Verification items for the finished model (mm, model axes). Coordinates: 2 decimals unless noted, no trailing zeros. Order: outer loops, then holes, each group sorted by start corner. A loop starts at its lowest first (then second) coordinate and runs counter-clockwise, first axis right, second up. Notation, with made-up numbers: M -23,25.25 L 17,25.25 A25 cw 17,56.25 Z; hole C -29,44.5 d8. An arc over 180 degrees is marked long. Return JSON: item names as keys, results as strings. Group by question number.
Q1. Go/stop test with flat-tipped pins: pin 1 Ø1 at (x, y) = (-16, -1) entering from -Z; pin 2 Ø0.8 at (y, z) = (0.5, -5) entering from +X; pin 3 Ø1 at (x, y) = (12.5, -0.5) entering from +Z. Record where each tip stops, or that it passes through.
Q2. Section check C-C, the plane x = 6. Enter the section's corners in (y, z), then the cut area to 3 significant figures.
Q3. Section check A-A, the plane z = -37. Enter the section's corners in (x, y) (3 decimals), then the cut area to 3 significant figures.
Q4. Section check B-B, the plane z = 33. Enter the section's corners in (x, y), then the cut area to 3 significant figures.
Q5. Thickness scan on probe 1 along X at (y, z) = (-0.6, -37) (3 decimals); probe 2 along Z at (x, y) = (-5, -0.9); probe 3 along Z at (x, y) = (-6.5, -0.9). Record the ranges inside material, lowest first.
Q6. Section check D-D, the plane y = -0.55. Count the separate pieces of the cut face and the enclosed holes in it, then the cut area to 3 significant figures.
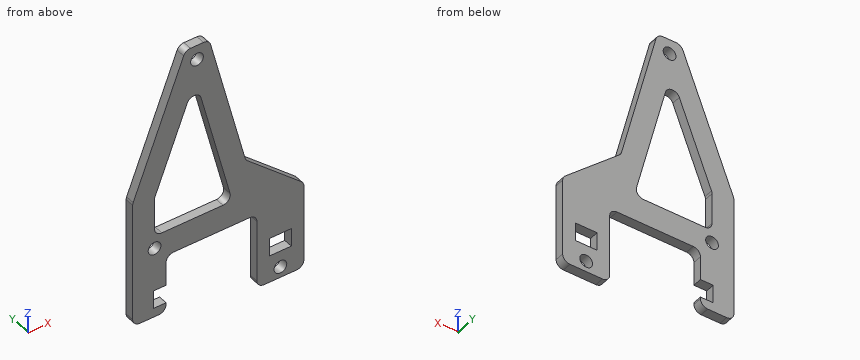
from build123d import *

# Parameters (mm, degrees)
BOSS_EXTRUDE1_DEPTH = 1.25
FILLET2_R           = 2
SKETCH2_R           = 1.75
SKETCH2_W           = 6
SKETCH2_H           = 5
SKETCH2_W_2         = 3.5
CUT_EXTRUDE1_DEPTH  = 48.430298597


with BuildPart() as part:
    # Sketch1 → Boss-Extrude1 (new, symmetric)
    with BuildSketch(Plane(origin=(0, 0, 0), x_dir=(1, 0, 0), z_dir=(0, 1, 0))):
        Polygon((-21.635, 0), (-21.635, 35), (-12.465, 35), (-12.465, 19), (12.465, 19), (12.465, 40), (25.365, 40), (25.365, 16), (9.365, 2), (-0.635, -37), (-7.135, -37), align=None)
        Polygon((-15.635, 12), (5.735003444, 12), (-4.401302874, -27.531594642), (-15.635, 1.133701473), align=None, mode=Mode.SUBTRACT)
    extrude(amount=BOSS_EXTRUDE1_DEPTH, both=True)

    # Fillet2
    fillet2_edges = [part.edges().sort_by_distance(p)[0] for p in [
        (-21.635, 0, 0),
        (-21.635, 0, -35),
        (-12.465, 0, -35),
        (-12.465, 0, -19),
        (12.465, 0, -19),
        (12.465, 0, -40),
        (25.365, 0, -40),
        (25.365, 0, -16),
        (9.365, 0, -2),
        (-0.635, 0, 37),
        (-7.135, 0, 37),
        (-15.635, 0, -12),
        (-15.635, 0, -1.133701473),
        (-4.401302874, 0, 27.531594642),
        (5.735003444, 0, -12),
    ]]
    fillet(fillet2_edges, radius=FILLET2_R)

    # Sketch2 → Cut-Extrude1 (cut, through all)
    with BuildSketch(Plane(origin=(0, 1.25, 0), x_dir=(1, 0, 0), z_dir=(0, 1, 0))):
        with Locations(Location((18.915, 37, 0), (0, 0, 270))):
            Circle(SKETCH2_R)
        with Locations(Location((-15.635, 15.5, 0), (0, 0, 270))):
            Circle(SKETCH2_R)
        with Locations(Location((-3.97878342, -33, 0), (0, 0, 270))):
            Circle(SKETCH2_R)
        with Locations((18.915, 30)):
            Rectangle(SKETCH2_W, SKETCH2_H)
        with Locations((-14.215, 30)):
            Rectangle(SKETCH2_W_2, SKETCH2_H)
    extrude(amount=-CUT_EXTRUDE1_DEPTH, mode=Mode.SUBTRACT)


solid = part.part
Numbers:
{
 "1": {"pin 1": "stops at z = -35", "pin 2": "stops at x = 13.25", "pin 3": "stops at z = -4.31"},
 "2": {"outline": "M -1.25,-19 L 1.25,-19 L 1.25,11.12 L -1.25,11.12 Z", "area": "75.3 mm2"},
 "3": {"outline": "M 12.465,-1.25 L 17.165,-1.25 L 17.165,1.25 L 12.465,1.25 Z; M 20.665,-1.25 L 25.365,-1.25 L 25.365,1.25 L 20.665,1.25 Z", "area": "23.5 mm2"},
 "4": {"outline": "M -8.7,-1.25 L -5.73,-1.25 L -5.73,1.25 L -8.7,1.25 Z; M -2.23,-1.25 L 0.39,-1.25 L 0.39,1.25 L -2.23,1.25 Z", "area": "14.0 mm2"},
 "5": {"probe 1": "x = 12.465 to 17.165, 20.665 to 25.365", "probe 2": "z = -19 to -12, 23.02 to 31.58, 34.42 to 37", "probe 3": "z = -19 to -12, 22.09 to 36.86"},
 "6": {"separate pieces": "1", "enclosed holes": "5", "area": "1,300 mm2"}
}
